Check sheet for the drawn part. Datum: minimum x, y, z corner. Units: mm. Give positions to 0.01 mm unless a question says otherwise; leave off trailing zeros. Loops run counter-clockwise (first coordinate to the right, second up) from the corner with the lowest first, then second, coordinate; pieces in that order, holes last.
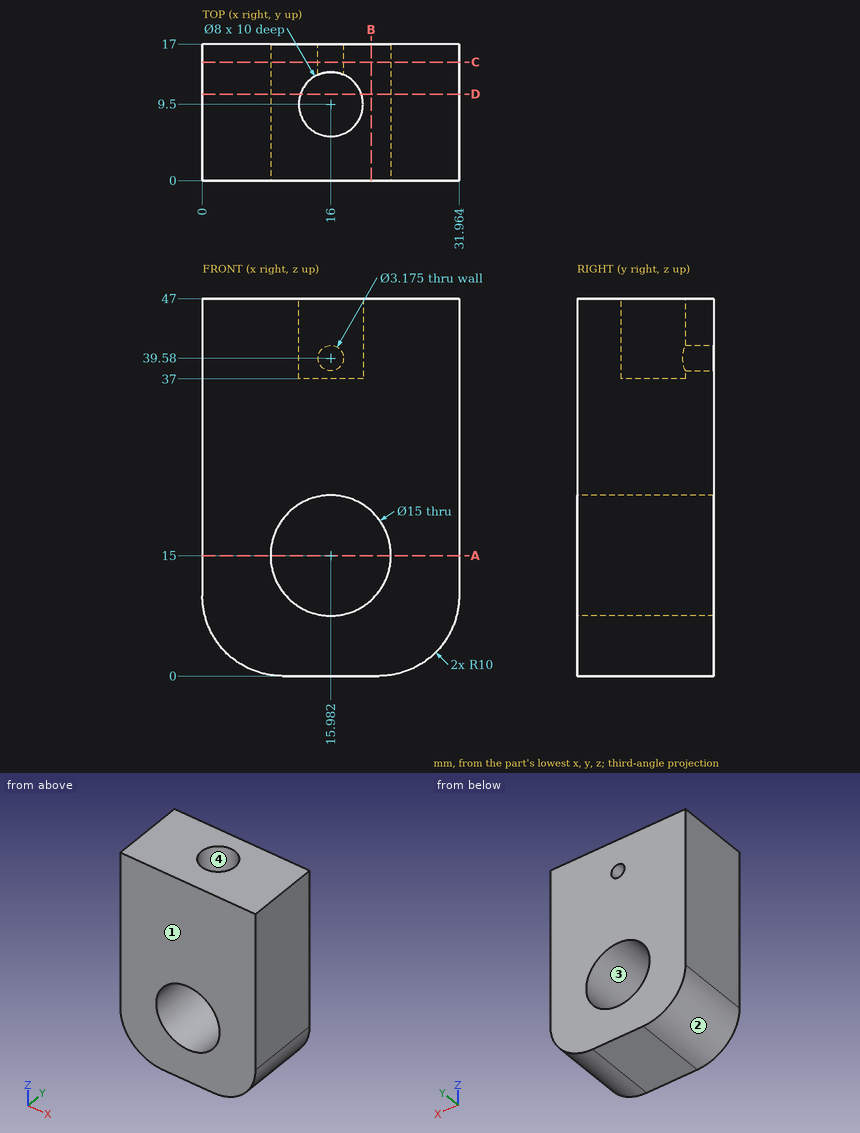
1) Scan lines: line 1 along X through (y, z) = (10.5, 15); line 2 along Z through (x, y) = (22, 1.5) (1 decimal); line 3 along X through (y, z) = (4.25, 11) (1 decimal). Record each from-to range of solid material in increasing order.
2) Mould release check, pull along X, two halves, no side actions. Record for the marked faces 1, 2, 3 and 4: +X half, -X half, draft (parallel to the pull), parting line (faces both ways), or undercut.
3) Sectioned sample at A-A on z = 15. Enter the section's corners in (x, y), plus the area to 3 significant figures.
4) Sectioned sample at D-D on y = 10.75. Enter the section's corners in (x, z).
5) Sectioned sample at C-C on y = 14.75. Enter the section's corners in (x, z) (1 decimal), plus the area to 3 significant figures.
6) Sectioned sample at B-B on x = 21. Enter the section's corners in (y, z).
Determined:
1. line 1: x = 0 to 8.48, 23.48 to 31.96
1. line 2: z = 0 to 10.5, 19.5 to 47
1. line 3: x = 0 to 9.6, 22.3 to 32
2. face 1: draft
2. face 2: -X half
2. face 3: undercut
2. face 4: undercut
3. outline: (0, 0) - (8.48, 0) - (8.48, 17) - (0, 17) - close; (23.48, 0) - (31.96, 0) - (31.96, 17) - (23.48, 17) - close
3. area: 288 mm2
4. outline: (0, 10) arc R10 ccw to (10, 0) - (21.96, 0) arc R10 ccw to (31.96, 10) - (31.96, 47) - (19.8, 47) - (19.8, 37) - (12.2, 37) - (12.2, 47) - (0, 47) - close; hole circle Ø15 at (15.98, 15)
5. outline: (0, 10) arc R10 ccw to (10, 0) - (22, 0) arc R10 ccw to (32, 10) - (32, 47) - (0, 47) - close; hole circle Ø15 at (16, 15); hole circle Ø3.2 at (16, 39.6)
5. area: 1,270 mm2
6. outline: (0, 0) - (17, 0) - (17, 9.43) - (0, 9.43) - close; (0, 20.57) - (17, 20.57) - (17, 47) - (0, 47) - close
